Here's how the part is built. I have some questions about the finished solid (model axes, mm). Round coordinates to 2 decimals unless told otherwise and drop trailing zeros. Order: outer loops, then holes, each group sorted by start corner. A loop starts at its lowest first (then second) coordinate and runs counter-clockwise, first axis right, second up. Notation, with made-up numbers: (-24, -27) -> (-20, -27) arc R18 cw to (-20, -12) -> close; hole circle Ø8 at (-35.75, -5.5). An arc over 180 degrees is marked (long way). Use a Markdown table: item, result. Add a question column.
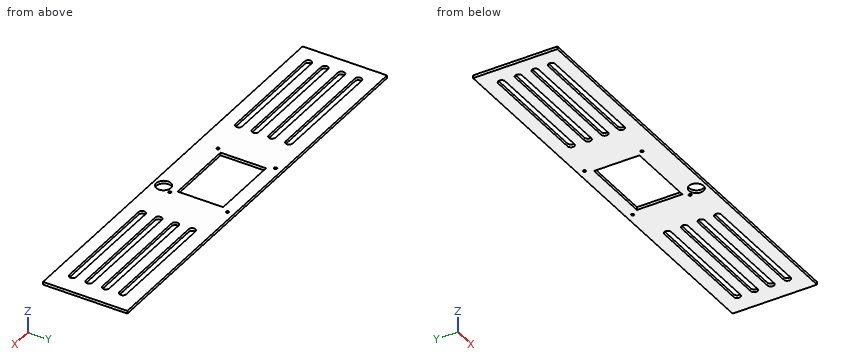
from build123d import *

# Parameters (mm, degrees)
SKETCH1_W           = 473.075
SKETCH1_H           = 95.25
BOSS_EXTRUDE1_DEPTH = 3.175
SKETCH3_W           = 78.74
SKETCH3_H           = 51.308
CUT_EXTRUDE2_DEPTH  = 242.305221983
SKETCH4_R           = 8.255
CUT_EXTRUDE3_DEPTH  = 242.305221983
SKETCH5_R           = 1.5875
CUT_EXTRUDE4_DEPTH  = 242.305221983
SKETCH6_W           = 3.175
SKETCH6_H           = 95.25
BOSS_EXTRUDE2_DEPTH = 371.948016105
SKETCH7_R           = 3.81
SKETCH7_W           = 50.8
SKETCH7_H           = 73.025
CUT_EXTRUDE5_DEPTH  = 381
CUT_EXTRUDE6_DEPTH  = 381
SKETCH12_W          = 371.948016105
SKETCH12_H          = 95.25
CUT_EXTRUDE7_DEPTH  = 54.356
SKETCH13_W          = 3.175
SKETCH13_H          = 95.25
BOSS_EXTRUDE3_DEPTH = 3.175


with BuildPart() as part:
    # Sketch1 → Boss-Extrude1 (new body)
    with BuildSketch(Plane.XY):
        Rectangle(SKETCH1_W, SKETCH1_H)
    extrude(amount=BOSS_EXTRUDE1_DEPTH)

    # Sketch3 → Cut-Extrude2 (cut, through all)
    with BuildSketch(Plane.XY.offset(3.175)):
        with Locations((0, 6.731)):
            Rectangle(SKETCH3_W, SKETCH3_H)
    extrude(amount=-CUT_EXTRUDE2_DEPTH, mode=Mode.SUBTRACT)

    # Sketch4 → Cut-Extrude3 (cut, through all)
    with BuildSketch(Plane.XY.offset(3.175)):
        with Locations((37.592, -35.814)):
            Circle(SKETCH4_R)
    extrude(amount=-CUT_EXTRUDE3_DEPTH, mode=Mode.SUBTRACT)

    # Sketch5 → Cut-Extrude4 (cut, through all)
    with BuildSketch(Plane.XY.offset(3.175)):
        with Locations((-44.196, 40.259)):
            Circle(SKETCH5_R)
        with Locations((44.196, 40.259)):
            Circle(SKETCH5_R)
        with Locations((-44.196, -24.765)):
            Circle(SKETCH5_R)
        with Locations((44.196, -24.765)):
            Circle(SKETCH5_R)
    extrude(amount=-CUT_EXTRUDE4_DEPTH, mode=Mode.SUBTRACT)

    # Sketch6 → Boss-Extrude2 (add)
    with BuildSketch(Plane(origin=(0, 0, 0), x_dir=(-1, 0, 0), z_dir=(0, 0, -1))):
        with Locations((234.95, 0)):
            Rectangle(SKETCH6_W, SKETCH6_H)
    extrude(amount=BOSS_EXTRUDE2_DEPTH)

    # Sketch7 → Cut-Extrude5 (cut)
    with BuildSketch(Plane.ZY.offset(236.5375)):
        with Locations((-248.250016105, -28.575)):
            Circle(SKETCH7_R)
        with Locations((-308.448016105, -7.9375)):
            Rectangle(SKETCH7_W, SKETCH7_H)
    extrude(amount=-CUT_EXTRUDE5_DEPTH, mode=Mode.SUBTRACT)

    # Sketch8 → Cut-Extrude6 (cut)
    with BuildSketch(Plane.XY.offset(3.175)):
        with BuildLine():
            Line((88.9, 31.75), (215.9, 31.75))
            ThreePointArc((215.9, 31.75), (219.71, 27.94), (215.9, 24.13))
            Line((215.9, 24.13), (88.9, 24.13))
            ThreePointArc((88.9, 24.13), (85.09, 27.94), (88.9, 31.75))
        make_face()
        with BuildLine():
            Line((88.9, 12.563594852), (215.9, 12.563594852))
            ThreePointArc((215.9, 12.563594852), (219.71, 8.753594852), (215.9, 4.943594852))
            Line((215.9, 4.943594852), (88.9, 4.943594852))
            ThreePointArc((88.9, 4.943594852), (85.09, 8.753594852), (88.9, 12.563594852))
        make_face()
        with BuildLine():
            Line((88.9, -6.256272006), (215.9, -6.256272006))
            ThreePointArc((215.9, -6.256272006), (219.71, -10.066272006), (215.9, -13.876272006))
            Line((215.9, -13.876272006), (88.9, -13.876272006))
            ThreePointArc((88.9, -13.876272006), (85.09, -10.066272006), (88.9, -6.256272006))
        make_face()
        with BuildLine():
            Line((88.9, -24.84600572), (215.9, -24.84600572))
            ThreePointArc((215.9, -24.84600572), (219.71, -28.65600572), (215.9, -32.46600572))
            Line((215.9, -32.46600572), (88.9, -32.46600572))
            ThreePointArc((88.9, -32.46600572), (85.09, -28.65600572), (88.9, -24.84600572))
        make_face()
        with BuildLine():
            Line((-88.9, -24.84600572), (-215.9, -24.84600572))
            ThreePointArc((-215.9, -24.84600572), (-219.71, -28.65600572), (-215.9, -32.46600572))
            Line((-215.9, -32.46600572), (-88.9, -32.46600572))
            ThreePointArc((-88.9, -32.46600572), (-85.09, -28.65600572), (-88.9, -24.84600572))
        make_face()
        with BuildLine():
            Line((-88.9, -6.256272006), (-215.9, -6.256272006))
            ThreePointArc((-215.9, -6.256272006), (-219.71, -10.066272006), (-215.9, -13.876272006))
            Line((-215.9, -13.876272006), (-88.9, -13.876272006))
            ThreePointArc((-88.9, -13.876272006), (-85.09, -10.066272006), (-88.9, -6.256272006))
        make_face()
        with BuildLine():
            Line((-88.9, 12.563594852), (-215.9, 12.563594852))
            ThreePointArc((-215.9, 12.563594852), (-219.71, 8.753594852), (-215.9, 4.943594852))
            Line((-215.9, 4.943594852), (-88.9, 4.943594852))
            ThreePointArc((-88.9, 4.943594852), (-85.09, 8.753594852), (-88.9, 12.563594852))
        make_face()
        with BuildLine():
            Line((-88.9, 31.75), (-215.9, 31.75))
            ThreePointArc((-215.9, 31.75), (-219.71, 27.94), (-215.9, 24.13))
            Line((-215.9, 24.13), (-88.9, 24.13))
            ThreePointArc((-88.9, 24.13), (-85.09, 27.94), (-88.9, 31.75))
        make_face()
    extrude(amount=-CUT_EXTRUDE6_DEPTH, mode=Mode.SUBTRACT)

    # Sketch12 → Cut-Extrude7 (cut)
    with BuildSketch(Plane(origin=(-233.3625, 0, 0), x_dir=(0, 0, -1), z_dir=(1, 0, 0))):
        with Locations((185.974008053, 0)):
            Rectangle(SKETCH12_W, SKETCH12_H)
    extrude(amount=-CUT_EXTRUDE7_DEPTH, mode=Mode.SUBTRACT)

    # Sketch13 → Boss-Extrude3 (add)
    with BuildSketch(Plane(origin=(236.5375, 0, 0), x_dir=(0, 0, -1), z_dir=(1, 0, 0))):
        with Locations((-1.5875, 0)):
            Rectangle(SKETCH13_W, SKETCH13_H)
    extrude(amount=BOSS_EXTRUDE3_DEPTH)


solid = part.part
(1) Please list where these lines run through material, in increasing order: probe 1 along Y at (x, z) = (-156, 2.9) (3 decimals); probe 2 along X at (y, z) = (14, 0.25); probe 3 along Y at (x, z) = (-4, 0.3) (3 decimals). Write a range as from..to.
(2) I want a section at B-B on z = 1.7. State how many separate pieces and enclosed holes the cut face has, and give its area (3 significant figures).
(3) I'm going to push a flat-ended pin straight in: P1, Ø1.9, axis at x = -44.196, y = 40.259, coming from the +Z side. Where does the tip first touch, or does it pass through?
(4) I want a section at A-A on x = -143. List the corners of the cut face in (y, z) for me (3 decimals).
Output:
| question | item | result |
|---|---|---|
| 1 | probe 1 | -47.625..-32.466, -24.846..-13.876, -6.256..4.944, 12.564..24.13, 31.75..47.625 |
| 1 | probe 2 | -236.54..-39.37, 39.37..239.71 |
| 1 | probe 3 | -47.625..-18.923, 32.385..47.625 |
| 2 | separate pieces | 1 |
| 2 | enclosed holes | 14 |
| 2 | area | 33,000 mm² |
| 3 | P1 | through |
| 4 | outline | (-47.625, 0) -> (-32.466, 0) -> (-32.466, 3.175) -> (-47.625, 3.175) -> close; (-24.846, 0) -> (-13.876, 0) -> (-13.876, 3.175) -> (-24.846, 3.175) -> close; (-6.256, 0) -> (4.944, 0) -> (4.944, 3.175) -> (-6.256, 3.175) -> close; (12.564, 0) -> (24.13, 0) -> (24.13, 3.175) -> (12.564, 3.175) -> close; (31.75, 0) -> (47.625, 0) -> (47.625, 3.175) -> (31.75, 3.175) -> close |
